from build123d import *

# Parameters (mm, degrees)
SKETCH_1_R      = 2.5
EXTRUDE_1_DEPTH = 240


with BuildPart() as part:
    # 草图1 → 凸台-拉伸1 (new body)
    with BuildSketch(Plane(origin=(0, 0, 0), x_dir=(1, 0, 0), z_dir=(0, 1, 0))):
        with BuildLine():
            Line((5.5, 8.2), (3.1, 8.201478584))
            Line((3.1, 8.201478584), (3.1, 9.5))
            Line((3.1, 9.5), (3.6, 10))
            Line((3.6, 10), (8.8, 10))
            ThreePointArc((8.8, 10), (9.648528137, 9.648528137), (10, 8.8))
            Line((10, 8.8), (10, 3.6))
            Line((10, 3.6), (9.5, 3.1))
            Line((9.5, 3.1), (8.201478584, 3.1))
            Line((8.201478584, 3.1), (8.2, 5.5))
            Line((8.2, 5.5), (6.5, 5.5))
            Line((6.5, 5.5), (3.9, 2.9))
            Line((3.9, 2.9), (3.9, -2.9))
            Line((3.9, -2.9), (6.5, -5.5))
            Line((6.5, -5.5), (8.2, -5.5))
            Line((8.2, -5.5), (8.201478584, -3.1))
            Line((8.201478584, -3.1), (9.5, -3.1))
            Line((9.5, -3.1), (10, -3.6))
            Line((10, -3.6), (10, -8.8))
            ThreePointArc((10, -8.8), (9.648528137, -9.648528137), (8.8, -10))
            Line((8.8, -10), (3.6, -10))
            Line((3.6, -10), (3.1, -9.5))
            Line((3.1, -9.5), (3.1, -8.201478584))
            Line((3.1, -8.201478584), (5.5, -8.2))
            Line((5.5, -8.2), (5.5, -6.5))
            Line((5.5, -6.5), (2.9, -3.9))
            Line((2.9, -3.9), (-2.9, -3.9))
            Line((-2.9, -3.9), (-5.5, -6.5))
            Line((-5.5, -6.5), (-5.5, -8.2))
            Line((-5.5, -8.2), (-3.1, -8.201478584))
            Line((-3.1, -8.201478584), (-3.1, -9.5))
            Line((-3.1, -9.5), (-3.6, -10))
            Line((-3.6, -10), (-8.8, -10))
            ThreePointArc((-8.8, -10), (-9.648528137, -9.648528137), (-10, -8.8))
            Line((-10, -8.8), (-10, -3.6))
            Line((-10, -3.6), (-9.5, -3.1))
            Line((-9.5, -3.1), (-8.201478584, -3.1))
            Line((-8.201478584, -3.1), (-8.2, -5.5))
            Line((-8.2, -5.5), (-6.5, -5.5))
            Line((-6.5, -5.5), (-3.9, -2.9))
            Line((-3.9, -2.9), (-3.9, 2.9))
            Line((-3.9, 2.9), (-6.5, 5.5))
            Line((-6.5, 5.5), (-8.2, 5.5))
            Line((-8.2, 5.5), (-8.201478584, 3.1))
            Line((-8.201478584, 3.1), (-9.5, 3.1))
            Line((-9.5, 3.1), (-10, 3.6))
            Line((-10, 3.6), (-10, 8.8))
            ThreePointArc((-10, 8.8), (-9.648528137, 9.648528137), (-8.8, 10))
            Line((-8.8, 10), (-3.6, 10))
            Line((-3.6, 10), (-3.1, 9.5))
            Line((-3.1, 9.5), (-3.1, 8.201478584))
            Line((-3.1, 8.201478584), (-5.5, 8.2))
            Line((-5.5, 8.2), (-5.5, 6.5))
            Line((-5.5, 6.5), (-2.9, 3.9))
            Line((-2.9, 3.9), (2.9, 3.9))
            Line((2.9, 3.9), (5.5, 6.5))
            Line((5.5, 6.5), (5.5, 8.2))
        make_face()
        with Locations(Location((0, 0, 0), (0, 0, 270))):
            Circle(SKETCH_1_R, mode=Mode.SUBTRACT)
    extrude(amount=EXTRUDE_1_DEPTH)


solid = part.part
For this review, take the finished solid that the model builds, in its own axes (mm). A direction names the side the tool comes from. Round coordinates to 2 decimals unless told otherwise and drop trailing zeros. Order: outer loops, then holes, each group sorted by start corner. A loop starts at its lowest first (then second) coordinate and runs counter-clockwise, first axis right, second up. Notation, with made-up numbers: (-9.75, -18.75) -> (12.25, -18.75) arc R22 cw to (12.25, 17.25) -> close; hole circle Ø1 at (55, -30). An arc over 180 degrees is marked (long way). Write item = value, one per line. Start each with the question number.
1) Tool access review of faces 1 (the face through (-3.9, 118, 0)), 2 (the face through (3.9, 118, 0)), 3 (the face through (0, 118, -3.9)): name each direction out of +Z, -Z, +X, -X, +Y, -Y from which nothing blocks a thin tool from reaching the whole face with its end or side.
2) Insertion check: pin 1 (1.7 mm diameter, centred on x = 0.5, y = 147, fed in from -Z); pin 2 (6 mm diameter, centred on x = 0, z = -7, fed in from +Y); pin 3 (1.7 mm diameter, centred on y = 176, z = -1.5, fed in from -X); pin 4 (1.7 mm diameter, centred on y = 107.5, z = 0.5, fed in from +X). Each pin has a flat end and moves straight along its axis. Give the tip position at first contact, or say it passes through.
3) The part is to be moulded in two halves that separate along X. For faces 4 (the face through (-10, 118, -6)), 5 (the face through (-2, 0, -2)), 6 (the face through (0, 118, 3.9)), say which applies: +X half, -X half, draft (parallel to the pull), parting line (faces both ways), or undercut.
4) Take a section at B-B on x = 0. State the section outline as (y, z) points, plus the area to 3 significant figures.
5) Take a section at A-A on z = 0. State the section outline as (x, y) points.
6) To check wall thickness, follow line 1 (Z direction, x = 7.5, y = 123); line 2 (Z direction, x = -4.75, y = 226); line 3 (X direction, y = 223.5, z = 4). State the ranges of each line that lie inside material, in increasing order. Write a range as from..to.
Verdict:
q1.face_1 = -X, +Y, -Y
q1.face_2 = +X, +Y, -Y
q1.face_3 = -Z, +Y, -Y
q2.pin_1 = -3.9
q2.pin_2 = through
q2.pin_3 = -3.9
q2.pin_4 = 3.9
q3.face_4 = -X half
q3.face_5 = draft
q3.face_6 = undercut
q4.outline = (0, -3.9) -> (240, -3.9) -> (240, -2.5) -> (0, -2.5) -> close; (0, 2.5) -> (240, 2.5) -> (240, 3.9) -> (0, 3.9) -> close
q4.area = 672 mm2
q5.outline = (-3.9, 0) -> (-2.5, 0) -> (-2.5, 240) -> (-3.9, 240) -> close; (2.5, 0) -> (3.9, 0) -> (3.9, 240) -> (2.5, 240) -> close
q6.line_1 = -10..-5.5, 5.5..10
q6.line_2 = -10..-8.2, -5.75..-3.75, 3.75..5.75, 8.2..10
q6.line_3 = -10..-8.2, -5..-3, 3..5, 8.2..10
